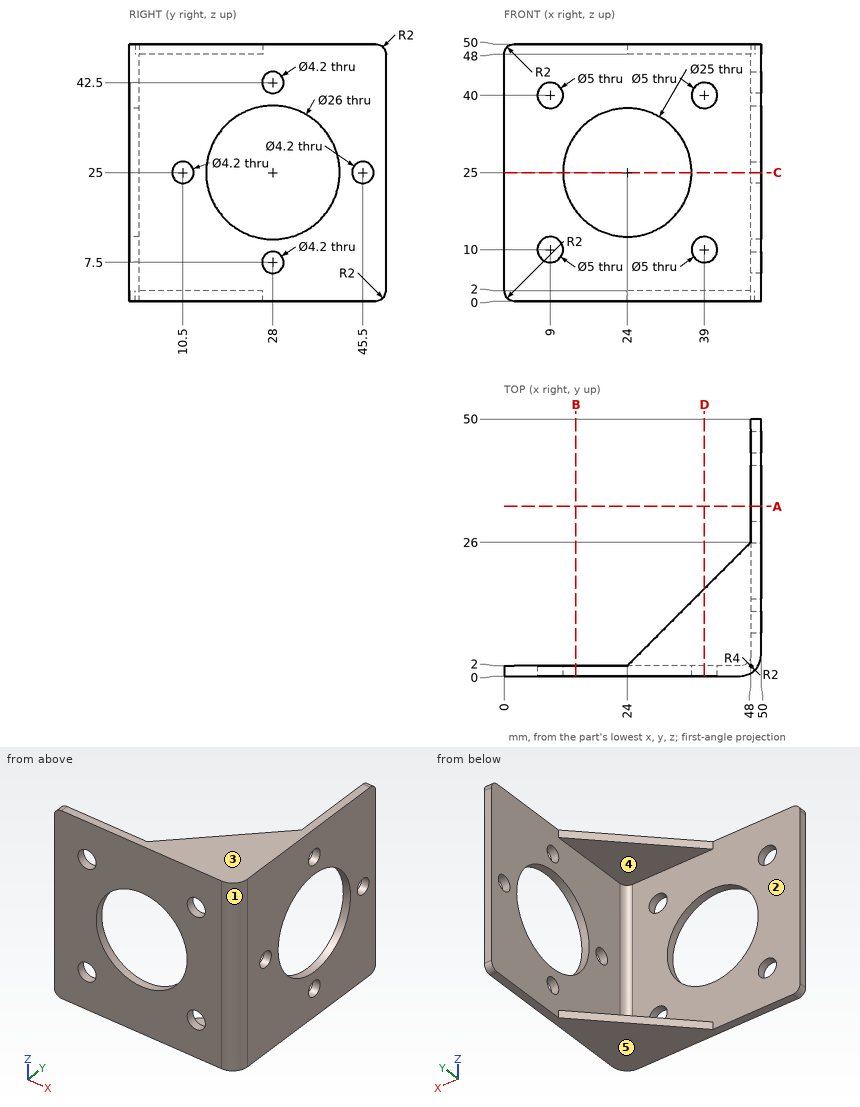
Answer from the drawing. Dimensions are ordinates in mm from the lowest x, y and z of the part. A direction names the side the tool comes from. Give positions to 0.01 mm unless a question says otherwise; leave off trailing zeros. Loops run counter-clockwise (first coordinate to the right, second up) from the corner with the lowest first, then second, coordinate; pieces in that order, holes last.
Item 1: A cutting plane is placed at B-B (x = 14). Give the vertices of the cut face in (y, z).
Derived:
outline: (0, 0) - (2, 0) - (2, 17.5) - (0, 17.5) - close; (0, 32.5) - (2, 32.5) - (2, 50) - (0, 50) - close
Item 2: A cutting plane is placed at A-A (y = 33). Give the vertices of the cut face in (x, z).
Derived:
outline: (48, 0) - (50, 0) - (50, 13) - (48, 13) - close; (48, 37) - (50, 37) - (50, 50) - (48, 50) - close
Item 3: A tool of negligible diameter and unlimited length cuts with its end or side. For the marked faces 4 and 5, from which of +Z, -Z, +X, -X, +Y, -Y can it reach the whole face along a straight path? Write none if from no direction.
Derived:
face 4: -X, +Y
face 5: -Z, +X, -X, +Y, -Y
Item 4: Determine the mould class of the marked faces 1, 2 and 3 for opening direction Z: +Z half, -Z half, draft (parallel to the pull), parting line (faces both ways), or undercut.
Derived:
face 1: draft
face 2: undercut
face 3: +Z half
Item 5: Each of these flat-tipped pins is pushed along its axis until it touches: pin 1 Ø6.5 at (x, z) = (9, 40) entering from +Y; pin 2 Ø1.5 at (y, z) = (43, 26) entering from -X. Where does it stop, or does it pass through?
Derived:
pin 1: stops at y = 2
pin 2: stops at x = 48
Item 6: Find the intervals of material crossed by line 1 along Z through (x, y) = (39, 1.05); line 2 along Y through (x, z) = (49, 25); line 3 along Z through (x, y) = (24, 1), in increasing order.
Derived:
line 1: z = 0 to 7.5, 12.5 to 37.5, 42.5 to 50
line 2: y = 1.35 to 8.4, 12.6 to 15, 41 to 43.4, 47.6 to 50
line 3: z = 0 to 12.5, 37.5 to 50
Item 7: A cutting plane is placed at C-C (z = 25). Give the vertices of the cut face in (x, y), then the cut area to 3 significant figures.
Derived:
outline: (0, 0) - (11.5, 0) - (11.5, 2) - (0, 2) - close; (36.5, 0) - (46, 0) arc R4 ccw to (50, 4) - (50, 8.4) - (48, 8.4) - (48, 4) arc R2 cw to (46, 2) - (36.5, 2) - close; (48, 12.6) - (50, 12.6) - (50, 15) - (48, 15) - close; (48, 41) - (50, 41) - (50, 43.4) - (48, 43.4) - close; (48, 47.6) - (50, 47.6) - (50, 50) - (48, 50) - close
area: 74.6 mm2
Item 8: A cutting plane is placed at D-D (x = 39). Give the vertices of the cut face in (y, z).
Derived:
outline: (0, 0) - (17, 0) - (17, 2) - (2, 2) - (2, 7.5) - (0, 7.5) - close; (0, 12.5) - (2, 12.5) - (2, 37.5) - (0, 37.5) - close; (0, 42.5) - (2, 42.5) - (2, 48) - (17, 48) - (17, 50) - (0, 50) - close
